Geometry: see drawing. Coordinates: mm, zero at the bounding-box minimum. Give positions to 0.01 mm unless a question says otherwise; leave off trailing zeros. Write each loop counter-clockwise with the first axis right and the second up, starting at its lowest first coordinate (ties: lowest second). Pieces come first, ordered by that corner, then holes. Notation, with made-up numbers: (4, 5.5) - (16, 5.5) arc R20 ccw to (16, 28.5) - close; hole circle Ø2 at (81.25, 32). An arc over 180 degrees is marked (long way). Answer as CSV lines item,"result". Start each with the question number.
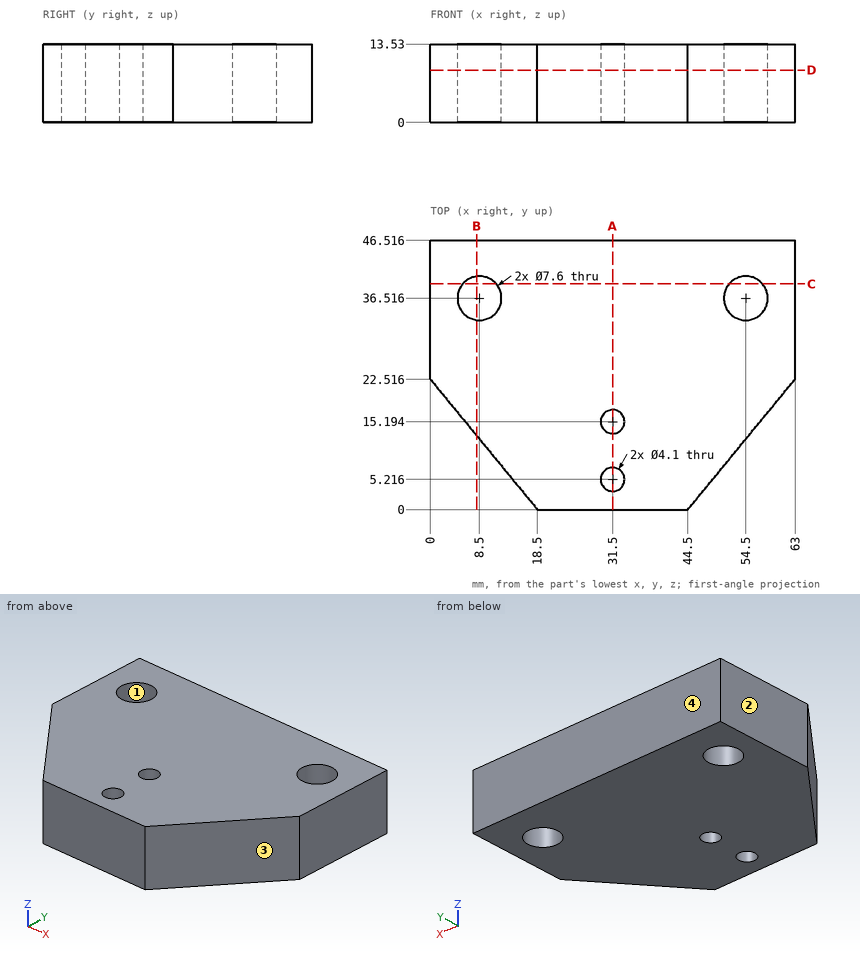
1) Pull-direction query (Y, two-part tool) for the marked faces 1, 2, 3 and 4; classes: +Y half, -Y half, draft (parallel to the pull), parting line (faces both ways), or undercut.
2) Material intervals for line 1 (Y direction, x = 31.5, z = 10.5) (1 decimal); line 2 (X direction, y = 38.5, z = 12.5); line 3 (X direction, y = 35, z = 7) (1 decimal), sorted ascending. Write a range as from..to.
3) Cut plane A-A on x = 31.5. Output: boundary loops of the cut face in (y, z) (1 decimal).
4) Cut plane B-B on x = 8. Output: boundary loops of the cut face in (y, z) (1 decimal).
5) Cut plane D-D on z = 9. State how many separate pieces and enclosed holes the cut face has, and give its area (3 significant figures).
6) Cut plane C-C on y = 39. Output: boundary loops of the cut face in (x, z) (1 decimal), and give its area (3 significant figures).
7) Contact query for flat-ended pins moving along their axis: P1, Ø3, axis at x = 53.5, y = 6, coming from the +Z side; P2, Ø1.5, axis at y = 6, z = 11.5, coming from the +X side (1 decimal); P3, Ø8, axis at x = 55.5, z = 4.5, coming from the -Y side; P4, Ø1, axis at x = 27, y = 7.5, coming from the -Z side. Output: stop coordinate, or through.
Numbers:
1,face 1,"undercut"
1,face 2,"draft"
1,face 3,"-Y half"
1,face 4,"+Y half"
2,line 1,"y = 0..3.2, 7.3..13.1, 17.2..46.5"
2,line 2,"x = 0..5.26, 11.74..51.26, 57.74..63"
2,line 3,"x = 0..5, 12..51, 58..63"
3,outline,"(0, 0) - (3.2, 0) - (3.2, 13.5) - (0, 13.5) - close; (7.3, 0) - (13.1, 0) - (13.1, 13.5) - (7.3, 13.5) - close; (17.2, 0) - (46.5, 0) - (46.5, 13.5) - (17.2, 13.5) - close"
4,outline,"(12.8, 0) - (32.7, 0) - (32.7, 13.5) - (12.8, 13.5) - close; (40.3, 0) - (46.5, 0) - (46.5, 13.5) - (40.3, 13.5) - close"
5,separate pieces,"1"
5,enclosed holes,"4"
5,area,"2,400 mm²"
6,outline,"(0, 0) - (5.6, 0) - (5.6, 13.5) - (0, 13.5) - close; (11.4, 0) - (51.6, 0) - (51.6, 13.5) - (11.4, 13.5) - close; (57.4, 0) - (63, 0) - (63, 13.5) - (57.4, 13.5) - close"
6,area,"697 mm²"
7,P1,"passes through"
7,P2,"stops at x = 50"
7,P3,"stops at y = 8.52"
7,P4,"stops at z = 0"
